The model under review builds one solid part; all positions refer to its coordinate system, in mm. A direction names the side the tool comes from. Coordinates: 2 decimals unless noted, no trailing zeros. Loops run counter-clockwise (first coordinate to the right, second up) from the corner with the lowest first, then second, coordinate; pieces in that order, holes last. Notation, with made-up numbers: (-1.5, 62.5) - (5.5, 62.5) arc R19 ccw to (5.5, 92.5) - close; hole circle Ø8 at (19.5, -29.75). An arc over 180 degrees is marked (long way). Use a Markdown table: item, result. Add a question column.
1) Clearance check with flat-ended pins moving along their axes: pin 1 (2 mm diameter, centred on x = 11.5, z = 4, fed in from +Y); pin 2 (0.5 mm diameter, centred on x = 14, z = 7.5, fed in from -Y); pin 3 (3 mm diameter, centred on y = 11.5, z = 5, fed in from -X); pin 4 (1.8 mm diameter, centred on x = 12.83, y = 57.87, fed in from +Z). State where each tip first meets the part, or that it passes through.
2) Add section B-B, the plane z = 1.5. Give the boundary of the cut face in (x, y).
3) Add section C-C, the plane x = -17. Give the boundary of the cut face in (y, z).
4) To check wall thickness, follow L1, parallel to Y at x = -20, z = 3; L2, parallel to X at y = -20, z = 3.25; L3, parallel to Y at x = 9.5, z = 0.5. State the ranges of each line that lie inside material, in increasing order. Write a range as [from, to].
5) For faces 4 (the flat face through (-11, -3.871, 4)), 5 (the flat face through (14, -2, 7)), 6 (the flat face through (14, -27.149, 3)), list the 3-axis set-ups (+Z, -Z, +X, -X, +Y, -Y) from which the entire face can be reached by the end or side of a thin tool; tool diameter is ignored.
6) Add section D-D, the plane y = 26. Give the boundary of the cut face in (x, z), and give its area (3 significant figures).
7) Add section A-A, the plane y = -18. Give the boundary of the cut face in (x, z).
8) The part is to be moulded in two halves that separate along Y. For faces 1 (the flat face through (0, -13, 8)), 2 (the flat face through (19.552, -16, 4)), 3 (the flat face through (21.787, 12.515, 3.944)), say which applies: pulls with the +Y half, pulls with the -Y half, needs draft (parallel to the pull), parting line crosses it, or undercut.
```python
from build123d import *

# Parameters (mm, degrees)
SKETCH1_R               = 1.5
BOSS_EXTRUDE1_DEPTH     = 8
CUT_EXTRUDE1_DEPTH      = 69.992355237
CUT_EXTRUDE1_DEPTH_BACK = 20
SKETCH2_R               = 2.25
SKETCH2_3_W             = 11.5
SKETCH2_3_H             = 5
CUT_EXTRUDE2_DEPTH      = 1


with BuildPart() as part:
    # Sketch1 → Boss-Extrude1 (new body)
    with BuildSketch(Plane.XY):
        with BuildLine():
            Line((18.829016979, 57.870689655), (24.829016979, -34.129310345))
            ThreePointArc((24.829016979, -34.129310345), (12.829016979, -46.129310345), (0.829016979, -34.129310345))
            Line((0.829016979, -34.129310345), (0.829016979, -63.870689655))
            Line((0.829016979, -63.870689655), (-24.829016979, -63.870689655))
            Line((-24.829016979, -63.870689655), (-24.829016979, -3.870689655))
            Line((-24.829016979, -3.870689655), (2.802405285, -3.870689655))
            Line((2.802405285, -3.870689655), (6.829016979, 57.870689655))
            ThreePointArc((6.829016979, 57.870689655), (12.829016979, 63.870689655), (18.829016979, 57.870689655))
        make_face()
        with Locations((12.829016979, 57.870689655)):
            Circle(SKETCH1_R, mode=Mode.SUBTRACT)
        with Locations((12.829016979, 14.570689655)):
            Circle(SKETCH1_R, mode=Mode.SUBTRACT)
    extrude(amount=BOSS_EXTRUDE1_DEPTH)

    # Sketch2 → Cut-Extrude1 (cut, two sides: drawn at the far end of the back side and taken through both)
    # profile 1 of 5: a face of its own
    with BuildSketch(Plane.XY.offset(8).offset(-CUT_EXTRUDE1_DEPTH_BACK)):
        with BuildLine():
            Line((19.552405285, -27.149310345), (19.552405285, -10.699310345))
            ThreePointArc((19.552405285, -10.699310345), (18.507945189, -14.003912319), (15.7540073, -16.107983895))
            ThreePointArc((15.7540073, -16.107983895), (13.802405285, -18.738530146), (11.850803269, -16.107983895))
            ThreePointArc((11.850803269, -16.107983895), (9.09686538, -14.003912319), (8.052405285, -10.699310345))
            Line((8.052405285, -10.699310345), (8.052405285, -27.149310345))
            Line((8.052405285, -27.149310345), (19.552405285, -27.149310345))
        make_face()
    # profile 2 of 5: a face of its own
    with BuildSketch(Plane.XY.offset(8).offset(-CUT_EXTRUDE1_DEPTH_BACK)):
        with BuildLine():
            ThreePointArc((15.7540073, -16.107983895), (13.802405285, -4.949310345), (11.850803269, -16.107983895))
            ThreePointArc((11.850803269, -16.107983895), (13.802405285, -18.738530146), (15.7540073, -16.107983895))
        make_face()
        with Locations((13.802405285, -10.699310345)):
            Circle(SKETCH2_R, mode=Mode.SUBTRACT)
    # profile 3 of 5: a face of its own
    with BuildSketch(Plane.XY.offset(8).offset(-CUT_EXTRUDE1_DEPTH_BACK)):
        with Locations((13.802405285, -10.699310345)):
            Circle(SKETCH2_R)
    # profile 4 of 5: a face of its own
    with BuildSketch(Plane.XY.offset(8).offset(-CUT_EXTRUDE1_DEPTH_BACK)):
        with BuildLine():
            Line((19.552405285, -4.949310345), (13.802405285, -4.949310345))
            ThreePointArc((13.802405285, -4.949310345), (17.868269276, -6.633446353), (19.552405285, -10.699310345))
            Line((19.552405285, -10.699310345), (19.552405285, -4.949310345))
        make_face()
    # profile 5 of 5: a face of its own
    with BuildSketch(Plane.XY.offset(8).offset(-CUT_EXTRUDE1_DEPTH_BACK)):
        with BuildLine():
            ThreePointArc((8.052405285, -10.699310345), (9.736541293, -6.633446353), (13.802405285, -4.949310345))
            Line((13.802405285, -4.949310345), (8.052405285, -4.949310345))
            Line((8.052405285, -4.949310345), (8.052405285, -10.699310345))
        make_face()
    extrude(amount=CUT_EXTRUDE1_DEPTH + CUT_EXTRUDE1_DEPTH_BACK, mode=Mode.SUBTRACT)

    # Sketch2_3 → Cut-Extrude2 (cut)
    with BuildSketch(Plane.XY.offset(8)):
        with Locations((13.802405285, -2.449310345)):
            Rectangle(SKETCH2_3_W, SKETCH2_3_H)
        with Locations((13.802405285, -29.649310345)):
            Rectangle(SKETCH2_3_W, SKETCH2_3_H)
    extrude(amount=-CUT_EXTRUDE2_DEPTH, mode=Mode.SUBTRACT)


solid = part.part
```
From the geometry:
| question | item | result |
|---|---|---|
| 1 | pin 1 | stops at y = 63.86 |
| 1 | pin 2 | stops at y = -46.09 |
| 1 | pin 3 | stops at x = 3.71 |
| 1 | pin 4 | passes through |
| 2 | outline | (-24.83, -63.87) - (0.83, -63.87) - (0.83, -34.13) arc R12 ccw to (24.83, -34.13) - (18.83, 57.87) arc R6 ccw to (6.83, 57.87) - (2.8, -3.87) - (-24.83, -3.87) - close; hole (8.05, -27.15) - (19.55, -27.15) - (19.55, -4.95) - (8.05, -4.95) - close; hole circle Ø3 at (12.83, 14.57); hole circle Ø3 at (12.83, 57.87) |
| 3 | outline | (-63.87, 0) - (-3.87, 0) - (-3.87, 8) - (-63.87, 8) - close |
| 4 | L1 | y = [-63.87, -3.87] |
| 4 | L2 | x = [-24.83, 8.05], [19.55, 23.91] |
| 4 | L3 | y = [-45.66, -27.15], [-4.95, 62.86] |
| 5 | face 4 | +Z, -Z, -X, +Y |
| 5 | face 5 | +Z |
| 5 | face 6 | +Z, -Z |
| 6 | outline | (4.75, 0) - (20.91, 0) - (20.91, 8) - (4.75, 8) - close |
| 6 | area | 129 mm^2 |
| 7 | outline | (-24.83, 0) - (8.05, 0) - (8.05, 8) - (-24.83, 8) - close; (19.55, 0) - (23.78, 0) - (23.78, 8) - (19.55, 8) - close |
| 8 | face 1 | needs draft |
| 8 | face 2 | undercut |
| 8 | face 3 | pulls with the +Y half |
